The model under review builds one solid part; all positions refer to its coordinate system, in mm. Face numbers are marked on the shaded views. A direction names the side the tool comes from. Round coordinates to 2 decimals unless told otherwise and drop trailing zeros. Return JSON: item names as keys, results as strings.
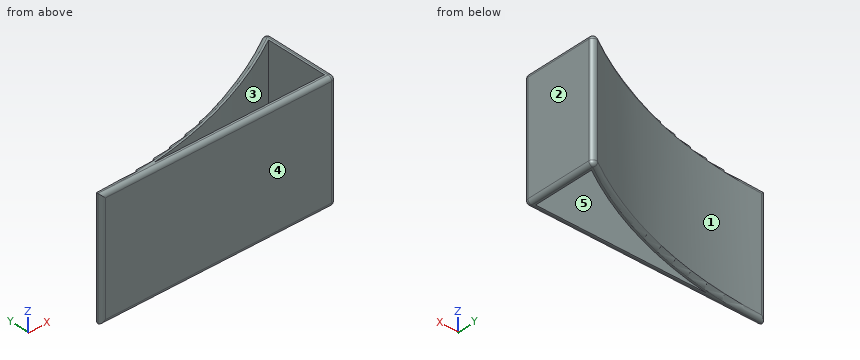
from build123d import *

# Parameters (mm, degrees)
F1_DEPTH = 30
F2_T     = -1.5
F3_R     = 0.99999


# Not quite as in the source:
# - a fillet or chamfer is up to 0.001 mm smaller than in the source, because OpenCascade refuses the exact size


with BuildPart() as f1:
    # F0 (on Top) → F1 (new body)
    with BuildSketch(Plane.XY):
        with BuildLine():
            Line((-60, 2), (-60, 0))
            Line((-60, 0), (0, 0))
            Line((0, 0), (0, 20))
            ThreePointArc((0, 20), (-28.6790804733, 6.5969349109), (-60, 2))
        make_face()
    extrude(amount=F1_DEPTH)

    # F2
    f2_openings = [f1.faces().sort_by_distance(p)[0] for p in [
        (-18.660264, 5.692192, 30),
        (-18.660264, 5.692192, 0),
    ]]
    offset(amount=F2_T, openings=f2_openings)

    # F3 (radius 1 in the source; OpenCascade refuses exactly that, so slightly less here)
    f3_edges = [f1.edges().sort_by_distance(p)[0] for p in [
        (-60, 2, 15),
        (-60, 0, 15),
        (-28.67908, 6.596935, 30),
        (-30, 0, 30),
        (-28.67908, 6.596935, 0),
        (-30, 0, 0),
        (0, 20, 15),
        (0, 0, 15),
        (0, 10, 30),
        (0, 10, 0),
    ]]
    fillet(f3_edges, radius=F3_R)


solid = f1.part
(1) Wall thickness on line 1 (X direction, y = 10.25, z = 7); line 2 (X direction, y = 12.75, z = 4.5); line 3 (Y direction, x = -27, z = 16.5): over which ranges is each line inside the solid? List them lowest first.
Filled in:
{"line 1": "x = -18.4 to -14.62, -1.5 to 0", "line 2": "x = -12.8 to -9.43, -1.5 to 0", "line 3": "y = 0 to 1.5, 5.54 to 7.12"}
(2) Mouldability with a two-part tool opening along Y and no side actions: class the marked faces 1, 2 and 3 as released by +Y, released by -Y, zero draft, split by the parting line, or undercut.
Filled in:
{"face 1": "released by +Y", "face 2": "zero draft", "face 3": "undercut"}
(3) Clearance check with flat-ended pins moving along their axes: pin 1 Ø4 at (y, z) = (13, 13) entering from -X; pin 2 Ø5 at (x, y) = (-7, 5.5) entering from -Z; pin 3 Ø3 at (y, z) = (15, 6) entering from -X. State where each tip first meets the part, or that it passes through.
Filled in:
{"pin 1": "stops at x = -16.63", "pin 2": "passes through", "pin 3": "stops at x = -11.27"}
(4) For the marked faces 4 and 5, list the 3-axis set-ups (+Z, -Z, +X, -X, +Y, -Y) from which the entire face can be reached by the end or side of a thin tool; tool diameter is ignored.
Filled in:
{"face 4": "+Z, -Z, +X, -X, -Y", "face 5": "+Z, -Z"}
